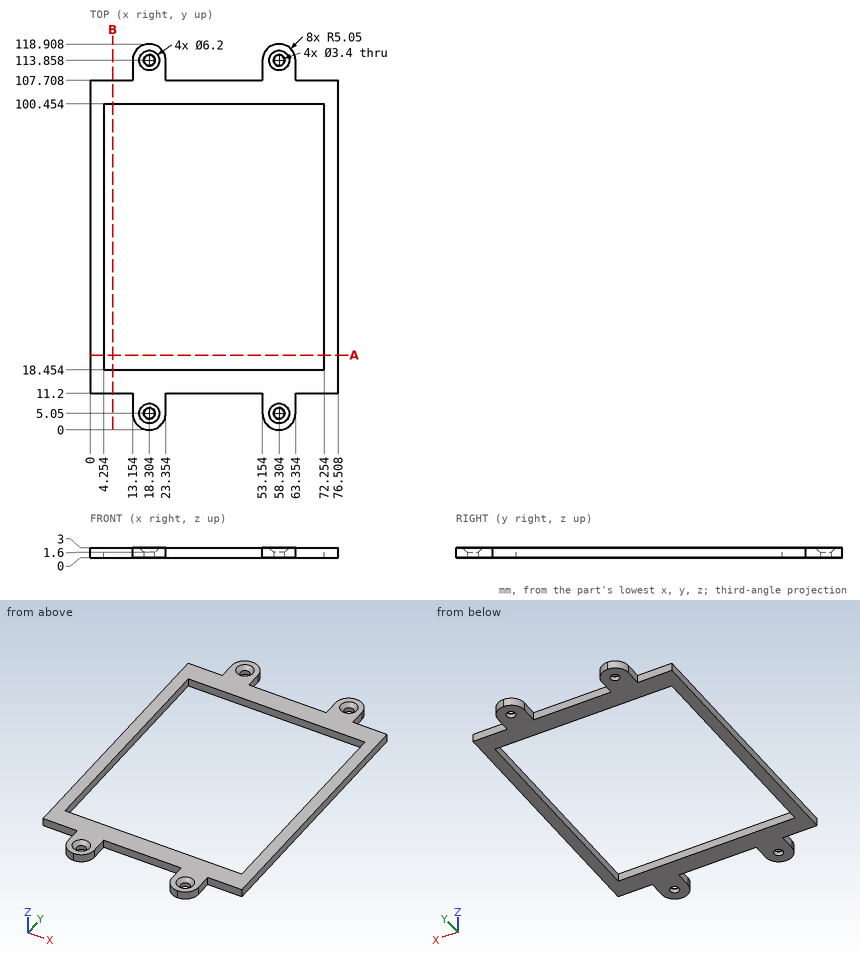
Could you check a few things on this drawing? It's one solid part, dimensions in mm from its lowest x, y, z. Give positions to 0.01 mm unless a question says otherwise; leave off trailing zeros. Loops run counter-clockwise (first coordinate to the right, second up) from the corner with the lowest first, then second, coordinate; pieces in that order, holes last. Notation, with made-up numbers: (57.5, -14.75) -> (93.5, -14.75) arc R24 ccw to (93.5, 7.25) -> close; hole circle Ø4 at (24.5, 5.25). An arc over 180 degrees is marked (long way). Answer as CSV lines item,"result". Start each with the question number.
(1) I need wall thicknesses on probe 1 along X at (y, z) = (5.05, 1.25); probe 2 along Y at (x, z) = (18.5, 0.8); probe 3 along Y at (x, z) = (44, 0.95). Which ranges of each line are inside material? Lowest first, please.
(2) If we section it at A-A on y = 23: Write out the boundary of the cut face in (x, z).
(3) If we section it at B-B on x = 7: Write out the boundary of the cut face in (y, z), then the cut area to 3 significant figures.
(4) I'm going to push flat-ended pins straight in: pin 1 Ø1.5 at (y, z) = (9, 2) entering from -X; pin 2 Ø0.9 at (y, z) = (8.5, 2) entering from +X; pin 3 Ø1.5 at (x, z) = (33.5, 1.5) entering from +Y. Where does each tip first touch, or does it pass through?
Computed:
1,probe 1,"x = 13.15 to 16.6, 20 to 23.35, 53.15 to 56.6, 60 to 63.35"
1,probe 2,"y = 0 to 3.36, 6.74 to 18.45, 100.45 to 112.17, 115.55 to 118.9"
1,probe 3,"y = 11.2 to 18.45, 100.45 to 107.71"
2,outline,"(0, 0) -> (4.25, 0) -> (4.25, 3) -> (0, 3) -> close; (72.25, 0) -> (76.51, 0) -> (76.51, 3) -> (72.25, 3) -> close"
3,outline,"(11.2, 0) -> (18.45, 0) -> (18.45, 3) -> (11.2, 3) -> close; (100.45, 0) -> (107.71, 0) -> (107.71, 3) -> (100.45, 3) -> close"
3,area,"43.5 mm2"
4,pin 1,"stops at x = 13.15"
4,pin 2,"stops at x = 63.35"
4,pin 3,"stops at y = 107.71"
